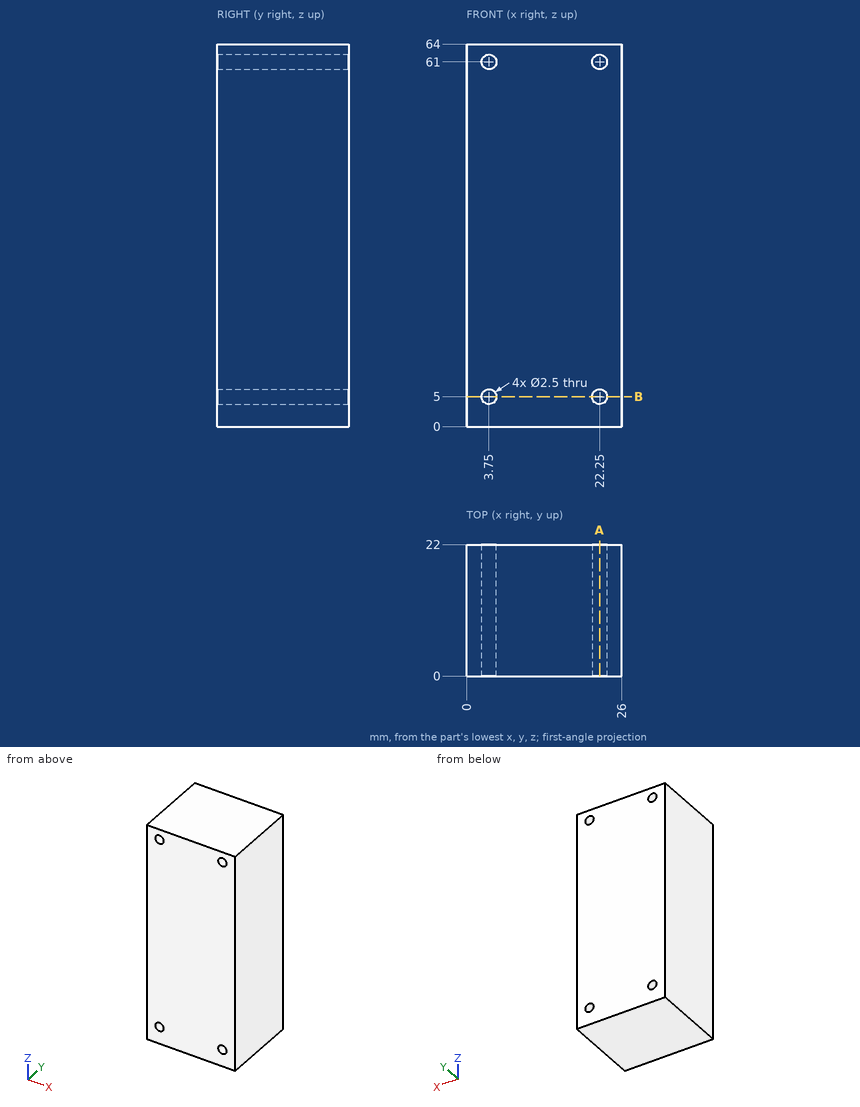
Job drawing, mm, ordinate dimensions from the low corner. One solid piece. Round coordinates to 2 decimals unless told otherwise and drop trailing zeros. Order: outer loops, then holes, each group sorted by start corner. A loop starts at its lowest first (then second) coordinate and runs counter-clockwise, first axis right, second up. Notation, with made-up numbers: (81.5, -35.75) - (128.5, -35.75) arc R13 cw to (128.5, -16.75) - close; hole circle Ø11 at (-5.75, 73). An arc over 180 degrees is marked (long way). Use CSV: the item, a comma, the result in double quotes. Start each with the question number.
1) Saw through at A-A (x = 22.25). List the corners of the cut face in (y, z), and give its area (3 significant figures).
2) Saw through at B-B (z = 5). List the corners of the cut face in (x, y).
3) Pin check, flat tip, straight feed: pin 1 Ø2 at (x, z) = (22.25, 5) entering from -Y. Stop position of the tip, or through.
4) Wall check: L1, parallel to Z at x = 22.25, y = 8.5; L2, parallel to X at y = 4, z = 60.5. Give the ranges that are in metal, low to high. Write a range as [from, to].
Values follow:
1,outline,"(0, 0) - (22, 0) - (22, 3.75) - (0, 3.75) - close; (0, 6.25) - (22, 6.25) - (22, 59.75) - (0, 59.75) - close; (0, 62.25) - (22, 62.25) - (22, 64) - (0, 64) - close"
1,area,"1,300 mm2"
2,outline,"(0, 0) - (2.5, 0) - (2.5, 22) - (0, 22) - close; (5, 0) - (21, 0) - (21, 22) - (5, 22) - close; (23.5, 0) - (26, 0) - (26, 22) - (23.5, 22) - close"
3,pin 1,"passes through"
4,L1,"z = [0, 3.75], [6.25, 59.75], [62.25, 64]"
4,L2,"x = [0, 2.6], [4.9, 21.1], [23.4, 26]"
